Autodesk Inventor part; units mm, degrees
ref_plane "YZ Plane" through (0, 0, 0) normal (1, 0, 0) x (0, 1, 0)
ref_plane "XZ Plane" through (0, 0, 0) normal (0, 1, 0) x (-1, 0, 0)
ref_plane "XY Plane" through (0, 0, 0) normal (0, 0, 1) x (1, 0, 0)
sketch "Sketch1" plane through (0, 0, 0) normal (0, 1, 0) x (-1, 0, 0)
  line L0 (0, 0) -> (20, 0)
  line L1 (20, 0) -> (20, -20)
  line L2 (20, -20) -> (0, -20)
  line L3 (0, -20) -> (0, 0)
  dimension "d0" = 20
  dimension "d1" = 20
extrude "Extrusion1" add sketch "Sketch1" along normal blind 3
sketch "Sketch2" plane through (0, 3, 0) normal (0, 1, 0) x (1, 0, 0)
  line L0 (0, 0) -> (-4, 0)
  line L1 (-4, 0) -> (-4, 4)
  line L2 (-4, 4) -> (0, 4)
  line L3 (0, 4) -> (0, 0)
  line L4 (0, 0) -> (-2, 0)
  line L5 (-2, 0) -> (-2, 2)
  line L6 (-2, 2) -> (0, 2)
  line L7 (0, 2) -> (0, 0)
  line L8 (0, 20) -> (-20, 20)
  line L9 (0, 20) -> (-4, 20)
  line L10 (-4, 20) -> (-4, 16)
  line L11 (-4, 16) -> (0, 16)
  line L12 (0, 16) -> (0, 20)
  line L13 (0, 20) -> (-2, 20)
  line L14 (-2, 20) -> (-2, 18)
  line L15 (-2, 18) -> (0, 18)
  line L16 (0, 18) -> (0, 20)
  line L17 (-20, 20) -> (-20, 0)
  line L18 (-20, 20) -> (-16, 20)
  line L19 (-16, 20) -> (-16, 16)
  line L20 (-16, 16) -> (-20, 16)
  line L21 (-20, 16) -> (-20, 20)
  line L22 (-20, 20) -> (-18, 20)
  line L23 (-18, 20) -> (-18, 18)
  line L24 (-18, 18) -> (-20, 18)
  line L25 (-20, 18) -> (-20, 20)
  line L26 (-20, 0) -> (-16, 0)
  line L27 (-16, 0) -> (-16, 4)
  line L28 (-16, 4) -> (-20, 4)
  line L29 (-20, 4) -> (-20, 0)
  line L30 (-20, 0) -> (-18, 0)
  line L31 (-18, 0) -> (-18, 2)
  line L32 (-18, 2) -> (-20, 2)
  line L33 (-20, 2) -> (-20, 0)
  circle A0 centre (-18, 2) radius 1
  circle A1 centre (-18, 18) radius 1
  circle A2 centre (-2, 2) radius 1
  circle A3 centre (-2, 18) radius 1
  dimension "d4" = 4
  dimension "d5" = 4
  dimension "d6" = 2
  dimension "d7" = 2
  dimension "d8" = 4
  dimension "d9" = 4
  dimension "d10" = 2
  dimension "d11" = 2
  dimension "d12" = 4
  dimension "d13" = 4
  dimension "d14" = 2
  dimension "d15" = 2
  dimension "d16" = 4
  dimension "d17" = 4
  dimension "d18" = 2
  dimension "d19" = 2
  dimension "d20" = 2
  dimension "d21" = 2
  dimension "d22" = 2
  dimension "d23" = 2
extrude "Extrusion2" add sketch "Sketch2" along normal blind 4 contours L0 L5 A2 L6 L3 | L0 L1 L2 L3 L6 A2 L5 | L12 L15 A3 L14 L8 | L19 L20 L17 L24 A1 L23 L8 | L14 A3 L15 L12 L11 L10 L8 | L23 A1 L24 L17 L8
properties part number "underplate_support_1"
For this review, take the finished solid that the model builds, in its own axes (mm). A direction names the side the tool comes from. Round coordinates to 2 decimals unless told otherwise and drop trailing zeros. Order: outer loops, then holes, each group sorted by start corner. A loop starts at its lowest first (then second) coordinate and runs counter-clockwise, first axis right, second up. Notation, with made-up numbers: M -20.5,79 L -8.5,79 A12 cw -8.5,89 Z; hole C 60,28.5 d9. An arc over 180 degrees is marked long. Use a Markdown table: item, result. Add a question column.
Item 1: Add section B-B, the plane x = -18. Give the boundary of the cut face in (y, z), then the cut area to 3 significant figures.
Item 2: Add section C-C, the plane z = -2. Give the boundary of the cut face in (x, y), then the cut area to 3 significant figures.
Item 3: Insertion check: pin 1 (2 mm diameter, centred on x = -2, z = -17.5, fed in from +Y); pin 2 (1 mm diameter, centred on x = -13.5, z = -13.5, fed in from +Y); pin 3 (1.5 mm diameter, centred on x = -8.5, y = 5, fed in from +Z); pin 4 (1.2 mm diameter, centred on x = -18.5, y = 4.5, fed in from +Z). Each pin has a flat end and moves straight along its axis. Give the tip position at first contact, or say it passes through.
Item 4: Tool access review of faces 4 (the flat face through (-18, 5, -16)), 5 (the flat face through (-16, 5, -18)), 6 (the flat face through (-2, 3, -18)): name each direction out of +Z, -Z, +X, -X, +Y, -Y from which nothing blocks a thin tool from reaching the whole face with its end or side.
Item 5: To check wall thickness, follow line 1 along X through (y, z) = (5.65, -18); line 2 along X through (y, z) = (4.05, -2). State the ranges of each line that lie inside material, in increasing order.
Item 6: Add section A-A, the plane y = 4. Give the boundary of the cut face in (x, z).
Item 7: Mouldability with a two-part tool opening along X and no side actions: class faces 1 (the flat face through (-20, 2, -12)), 2 (the flat face through (-2, 5, -16)), 3 (the cylindrical face through (-18, 5, -19)) as released by +X, released by -X, zero draft, split by the parting line, or undercut.
Item 8: Add section D-D, the plane x = -2. Give the boundary of the cut face in (y, z).
Geometry results:
| question | item | result |
|---|---|---|
| 1 | outline | M 0,-20 L 7,-20 L 7,-19 L 3,-19 L 3,-17 L 7,-17 L 7,-16 L 3,-16 L 3,0 L 0,0 Z |
| 1 | area | 68.0 mm² |
| 2 | outline | M -20,0 L 0,0 L 0,7 L -1,7 L -1,3 L -3,3 L -3,7 L -4,7 L -4,3 L -20,3 Z |
| 2 | area | 68.0 mm² |
| 3 | pin 1 | stops at y = 7 |
| 3 | pin 2 | stops at y = 3 |
| 3 | pin 3 | passes through |
| 3 | pin 4 | stops at z = -16 |
| 4 | face 4 | +Z, +X, -X, +Y |
| 4 | face 5 | +Z, -Z, +Y |
| 4 | face 6 | +Y |
| 5 | line 1 | x = -20 to -19, -17 to -16, -4 to -3, -1 to 0 |
| 5 | line 2 | x = -4 to -3, -1 to 0 |
| 6 | outline | M -20,-20 L -16,-20 L -16,-16 L -20,-16 Z; M -4,-20 L 0,-20 L 0,-16 L -4,-16 Z; M -4,-4 L 0,-4 L 0,0 L -4,0 Z; hole C -18,-18 d2; hole C -2,-18 d2; hole C -2,-2 d2 |
| 7 | face 1 | released by -X |
| 7 | face 2 | zero draft |
| 7 | face 3 | undercut |
| 8 | outline | M 0,-20 L 7,-20 L 7,-19 L 3,-19 L 3,-17 L 7,-17 L 7,-16 L 3,-16 L 3,-4 L 7,-4 L 7,-3 L 3,-3 L 3,-1 L 7,-1 L 7,0 L 0,0 Z |
